Autodesk Inventor part; units mm, degrees
ref_plane "Work Plane4" through (-27.5, -67.5, 0) normal (0, 0, -1) x (0, 1, 0)
ref_plane "Work Plane5" through (-27.5, -67.5, -58.6068) normal (0, 0, 1) x (1, 0, 0)
ref_plane "YZ Plane" through (0, 0, 0) normal (1, 0, 0) x (0, 1, 0)
sketch "Sketch1" plane through (0, 0, 0) normal (0, 0, 1) x (1, 0, 0)
  line L0 (0, 95.9497) -> (0, -95.9497) construction
  line L1 (-39.9497, 0) -> (39.9497, 0) construction
  arc A0 (22.5, -67.5) -> (27.5, -62.5) centre (22.5, -62.5) ccw
  line L2 (27.5, -62.5) -> (27.5, 62.5)
  arc A1 (27.5, 62.5) -> (22.5, 67.5) centre (22.5, 62.5) ccw
  line L3 (22.5, 67.5) -> (-22.5, 67.5)
  arc A2 (-22.5, 67.5) -> (-27.5, 62.5) centre (-22.5, 62.5) ccw
  line L4 (-27.5, 62.5) -> (-27.5, -62.5)
  arc A3 (-27.5, -62.5) -> (-22.5, -67.5) centre (-22.5, -62.5) ccw
  line L5 (-22.5, -67.5) -> (22.5, -67.5)
  line L6 (24.5, 62.5) -> (24.5, -62.5)
  arc A4 (22.5, -64.5) -> (24.5, -62.5) centre (22.5, -62.5) ccw
  line L7 (22.5, -64.5) -> (-22.5, -64.5)
  arc A5 (-24.5, -62.5) -> (-22.5, -64.5) centre (-22.5, -62.5) ccw
  line L8 (-24.5, -62.5) -> (-24.5, 62.5)
  arc A6 (-22.5, 64.5) -> (-24.5, 62.5) centre (-22.5, 62.5) ccw
  line L9 (-22.5, 64.5) -> (22.5, 64.5)
  arc A7 (24.5, 62.5) -> (22.5, 64.5) centre (22.5, 62.5) ccw
  circle A8 centre (20.5, 60.5) radius 2.5 construction
  line L10 (20.5, 58) -> (24.5, 58)
  line L11 (18, 60.5) -> (18, 64.5)
  line L12 (22.9495, 60) -> (24.5, 60)
  line L13 (20, 62.9495) -> (20, 64.5)
  circle A9 centre (20.5, 60.5) radius 1.5
  arc A10 (22.9495, 60) -> (20, 62.9495) centre (20.5, 60.5) ccw
  arc A11 (18, 60.5) -> (20.5, 58) centre (20.5, 60.5) ccw
  circle A12 centre (20.5, -60.5) radius 2.5 construction
  line L14 (20.5, -58) -> (24.5, -58)
  line L15 (18, -60.5) -> (18, -64.5)
  line L16 (22.9495, -60) -> (24.5, -60)
  line L17 (20, -62.9495) -> (20, -64.5)
  circle A13 centre (20.5, -60.5) radius 1.5
  arc A14 (20, -62.9495) -> (22.9495, -60) centre (20.5, -60.5) ccw
  arc A15 (20.5, -58) -> (18, -60.5) centre (20.5, -60.5) ccw
  circle A16 centre (-20.5, 60.5) radius 2.5 construction
  line L18 (-20.5, 58) -> (-24.5, 58)
  line L19 (-18, 60.5) -> (-18, 64.5)
  line L20 (-22.9495, 60) -> (-24.5, 60)
  line L21 (-20, 62.9495) -> (-20, 64.5)
  circle A17 centre (-20.5, 60.5) radius 1.5
  arc A18 (-20, 62.9495) -> (-22.9495, 60) centre (-20.5, 60.5) ccw
  arc A19 (-20.5, 58) -> (-18, 60.5) centre (-20.5, 60.5) ccw
  line L22 (-20.5, -58) -> (-24.5, -58)
  arc A20 (-18, -60.5) -> (-20.5, -58) centre (-20.5, -60.5) ccw
  line L23 (-22.9495, -60) -> (-24.5, -60)
  circle A21 centre (-20.5, -60.5) radius 1.5
  line L24 (-18, -60.5) -> (-18, -64.5)
  circle A22 centre (-20.5, -60.5) radius 2.5 construction
  arc A23 (-22.9495, -60) -> (-20, -62.9495) centre (-20.5, -60.5) ccw
  line L25 (-20, -62.9495) -> (-20, -64.5)
  line L26 (-24.5, 60) -> (-24.5, 58)
  line L27 (-20, 64.5) -> (-18, 64.5)
  line L28 (24.5, -58) -> (24.5, -60)
  line L29 (18, -64.5) -> (20, -64.5)
  line L30 (-20, -64.5) -> (-18, -64.5)
  line L31 (-24.5, -58) -> (-24.5, -60)
  point P0 (-22.5, -62.5)
  point P1 (-22.5, 62.5)
  dimension "d6" = 3
  dimension "d7" = 5
  dimension "d8" = 7
  dimension "d9" = 7
  dimension "d10" = 2
  dimension "d11" = 2
  dimension "d12" = 3
  dimension "d20" = 55
  dimension "d21" = 135
  dimension "d22" = 5
ref_plane "Work Plane4" through (-27.5, -67.5, 0) normal (0, 0, -1) x (0, 1, 0)
ref_plane "Work Plane5" through (-27.5, -67.5, -58.6068) normal (0, 0, 1) x (1, 0, 0)
extrude "Extrusion1" add sketch "Sketch1" against normal blind 38.75 contours L5 A3 L4 A2 L3 A1 L2 A0 | L6 L10 A11 L11 L9 L13 A10 L12 | L6 L16 A14 L17 L7 L15 A15 L14 | L19 A19 L18 L8 L20 A18 L21 L9 | L7 L25 A23 L23 L8 L22 A20 L24
ref_plane "PLan support PowerPCB" through (0, 0, -2.7) normal (0, 0, 1) x (1, 0, 0)
sketch "Sketch2" plane through (0, 0, -2.7) normal (0, 0, 1) x (1, 0, 0)
  line L0 (24.5, 58) -> (24.5, -58)
  line L1 (22.5, 58) -> (22.5, -58)
  line L2 (24.5, 58) -> (22.5, 58)
  line L3 (24.5, -58) -> (22.5, -58)
  line L4 (0, 94.5) -> (0, -94.5) construction
  line L5 (-24.5, 58) -> (-24.5, -58)
  line L6 (-22.5, 58) -> (-22.5, -58)
  line L7 (-24.5, 58) -> (-22.5, 58)
  line L8 (-24.5, -58) -> (-22.5, -58)
  point P0 (0, 0)
  dimension "d15" = 2
extrude "Extrusion2" add sketch "Sketch2" against normal blind 2.5
fillet "Fillet1" radius 2 2 edges at (-22.5, 0, -5.2) (22.5, 0, -5.2)
equation "\"d9\" = d8"
equation "\"d11\" = d10"
equation "\"d13\" = -Top_Plate_Bottom_to_PowerPcb_Bottom"
equation "\"Plate_thickness\" = 3"
equation "\"Top_Plate_Bottom_to_PowerPcb_Bottom\" = 2.7"
properties part number "Box_Body" material "ABS Plastic"
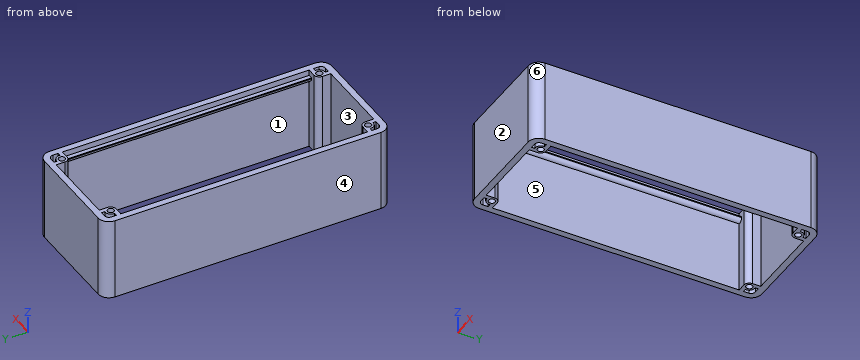
Verification items for the finished model (mm, model axes). Face numbers are marked on the shaded views. A direction names the side the tool comes from. Coordinates: 2 decimals unless noted, no trailing zeros. Order: outer loops, then holes, each group sorted by start corner. A loop starts at its lowest first (then second) coordinate and runs counter-clockwise, first axis right, second up. Notation, with made-up numbers: (85, 20.25) -> (132, 20.25) arc R20 ccw to (132, 55.25) -> close; hole circle Ø5 at (-29.5, 50). An arc over 180 degrees is marked (long way). Put each result on its own line as item: value. Start each with the question number.
1) Tool access check on the marked faces 1, 2 and 3. Record the directions out of +Z, -Z, +X, -X, +Y, -Y that give a thin tool (end or side, any length) a straight path to the whole face; none if there is none.
2) Cross-section at A-A (x = -14.5). Enter the section's corners in (y, z), plus the area to 4 significant figures.
3) Cross-section at C-C (z = -12). State how many separate pieces and enclosed holes the cut face has, plus the area to 3 significant figures.
4) Go/stop test with flat-tipped pins: pin 1 (1.7 mm diameter, centred on y = -63.5, z = -22.5, fed in from -X); pin 2 (0.5 mm diameter, centred on x = -24, z = -24.5, fed in from +Y); pin 3 (0.8 mm diameter, centred on x = 23.5, z = -19.5, fed in from +Y). Record where each tip stops, or that it passes through.
5) Release check for a two-part mould opening along Y. For the marked faces 4, 5 and 6 record: pulls with the +Y half, pulls with the -Y half, needs draft (parallel to the pull), parting line crosses it, or undercut.
6) Material ranges on L1, parallel to Y at x = 20.5, z = -13.5; L2, parallel to X at y = 31, z = -19; L3, parallel to Y at x = -11, z = -21.5, recorded low to high.
Geometry check:
1. face 1: -Z
1. face 2: +Z, -Z, +X, -X, -Y
1. face 3: +Z, -Z
2. outline: (-67.5, -38.75) -> (-64.5, -38.75) -> (-64.5, 0) -> (-67.5, 0) -> close; (64.5, -38.75) -> (67.5, -38.75) -> (67.5, 0) -> (64.5, 0) -> close
2. area: 232.5 mm^2
3. separate pieces: 1
3. enclosed holes: 9
3. area: 1,170 mm^2
4. pin 1: stops at x = -27.5
4. pin 2: stops at y = 67.34
4. pin 3: stops at y = 67.46
5. face 4: needs draft
5. face 5: undercut
5. face 6: pulls with the -Y half
6. L1: y = -67.5 to -64.5, -63 to -62, -59 to -58, 58 to 59, 62 to 63, 64.5 to 67.5
6. L2: x = -27.5 to -24.5, 24.5 to 27.5
6. L3: y = -67.5 to -64.5, 64.5 to 67.5
